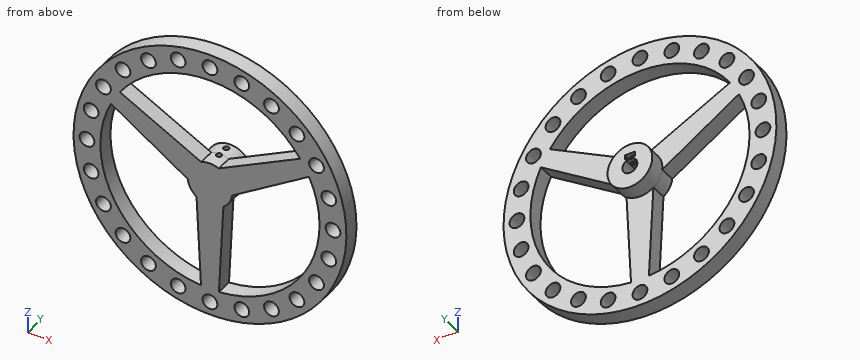
```python
from build123d import *
from build123d.topology import SkipClean

# Parameters (mm, degrees)
SKETCH1_R                      = 76.2
BOSS_EXTRUDE1_DEPTH            = 9
SKETCH2_R                      = 12.5
BOSS_EXTRUDE2_DEPTH            = 9
CUT_EXTRUDE1_DEPTH             = 13
CUT_EXTRUDE2_START             = -1
CUT_EXTRUDE2_DEPTH             = 2.5
CUT_EXTRUDE3_REACH             = 116.376
SKETCH5_R                      = 1.5
CUT_EXTRUDE3_DIRECTION_2_REACH = 116.376
SKETCH6_W                      = 5.5
SKETCH6_H                      = 2.5
CUT_EXTRUDE4_DEPTH             = 109.188743625
SKETCH7_R                      = 4.125
CUT_EXTRUDE5_DEPTH             = 109.138244862
CIRPATTERN1_COUNT              = 24


with BuildPart() as part:
    # Sketch1 → Boss-Extrude1 (new body)
    with BuildSketch(Plane(origin=(0, 0, 0), x_dir=(1, 0, 0), z_dir=(0, 1, 0))):
        with Locations(Location((0, 0, 0), (0, 0, 270))):
            Circle(SKETCH1_R)
        with BuildLine():
            Line((-7.5, 10), (-5, 60.995409663))
            ThreePointArc((-5, 60.995409663), (-53.000754712, 30.6), (-55.323574283, -26.167577813))
            Line((-55.323574283, -26.167577813), (-12.410254038, 1.495190528))
            ThreePointArc((-12.410254038, 1.495190528), (-10.825317547, 6.25), (-7.5, 10))
        make_face(mode=Mode.SUBTRACT)
        with BuildLine():
            Line((5, 60.995409663), (7.5, 10))
            ThreePointArc((7.5, 10), (10.825317547, 6.25), (12.410254038, 1.495190528))
            Line((12.410254038, 1.495190528), (55.323574283, -26.167577813))
            ThreePointArc((55.323574283, -26.167577813), (53.000754712, 30.6), (5, 60.995409663))
        make_face(mode=Mode.SUBTRACT)
        with BuildLine():
            Line((50.323574283, -34.827831851), (4.910254038, -11.495190528))
            ThreePointArc((4.910254038, -11.495190528), (0, -12.5), (-4.910254038, -11.495190528))
            Line((-4.910254038, -11.495190528), (-50.323574283, -34.827831851))
            ThreePointArc((-50.323574283, -34.827831851), (0, -61.2), (50.323574283, -34.827831851))
        make_face(mode=Mode.SUBTRACT)
    extrude(amount=BOSS_EXTRUDE1_DEPTH)

    # Sketch2 → Boss-Extrude2 (add)
    with BuildSketch(Plane(origin=(0, 9, 0), x_dir=(1, 0, 0), z_dir=(0, 1, 0))):
        with Locations(Location((0, 0, 0), (0, 0, 126.869897646))):
            Circle(SKETCH2_R)
    extrude(amount=BOSS_EXTRUDE2_DEPTH)

    # Sketch3 → Cut-Extrude1 (cut)
    with BuildSketch(Plane.XZ.offset(-18)):
        with BuildLine():
            Line((-1.981161276, 3.675), (1.981161276, 3.675))
            ThreePointArc((1.981161276, 3.675), (0, -4.175), (-1.981161276, 3.675))
        make_face()
    extrude(amount=CUT_EXTRUDE1_DEPTH, mode=Mode.SUBTRACT)

    # Sketch4 → Cut-Extrude2 (cut)
    with BuildSketch(Plane(origin=(0, 0, 3.675), x_dir=(-1, 0, 0), z_dir=(0, 0, -1)).offset(CUT_EXTRUDE2_START)):
        Polygon((0, 11.175426481), (-2.75, 9.58771324), (-2.75, 6.41228676), (0, 4.824573519), (2.75, 6.41228676), (2.75, 9.58771324), align=None)
    extrude(amount=-CUT_EXTRUDE2_DEPTH, mode=Mode.SUBTRACT)

    # Sketch5 → Cut-Extrude3 (cut, up to next)
    with BuildSketch(Plane(origin=(0, 0, 7.175), x_dir=(-1, 0, 0), z_dir=(0, 0, -1)), mode=Mode.PRIVATE) as cut_extrude3_sk1:
        with Locations((0, 8)):
            Circle(SKETCH5_R)
    cut_extrude3_tool1 = extrude(cut_extrude3_sk1.sketch, amount=-CUT_EXTRUDE3_REACH, mode=Mode.PRIVATE) & part.part
    # Sketch5 → Cut-Extrude3 (cut, up to next)
    with BuildSketch(Plane(origin=(0, 0, 7.175), x_dir=(-1, 0, 0), z_dir=(0, 0, -1)), mode=Mode.PRIVATE) as cut_extrude3_sk2:
        with Locations((0, 14.5)):
            Circle(SKETCH5_R)
    cut_extrude3_tool2 = extrude(cut_extrude3_sk2.sketch, amount=-CUT_EXTRUDE3_REACH, mode=Mode.PRIVATE) & part.part
    add(cut_extrude3_tool1.solids().sort_by_distance((0, 8, 7.175))[0], mode=Mode.SUBTRACT)
    add(cut_extrude3_tool2.solids().sort_by_distance((0, 14.5, 7.175))[0], mode=Mode.SUBTRACT)

    # Sketch5 → Cut-Extrude3 direction 2 (cut, up to next)
    with BuildSketch(Plane(origin=(0, 0, 7.175), x_dir=(-1, 0, 0), z_dir=(0, 0, -1)), mode=Mode.PRIVATE) as cut_extrude3_direction_2_sk1:
        with Locations((0, 8)):
            Circle(SKETCH5_R)
    cut_extrude3_direction_2_tool1 = extrude(cut_extrude3_direction_2_sk1.sketch, amount=CUT_EXTRUDE3_DIRECTION_2_REACH, mode=Mode.PRIVATE) & part.part
    # Sketch5 → Cut-Extrude3 direction 2 (cut, up to next)
    with BuildSketch(Plane(origin=(0, 0, 7.175), x_dir=(-1, 0, 0), z_dir=(0, 0, -1)), mode=Mode.PRIVATE) as cut_extrude3_direction_2_sk2:
        with Locations((0, 14.5)):
            Circle(SKETCH5_R)
    cut_extrude3_direction_2_tool2 = extrude(cut_extrude3_direction_2_sk2.sketch, amount=CUT_EXTRUDE3_DIRECTION_2_REACH, mode=Mode.PRIVATE) & part.part
    add(cut_extrude3_direction_2_tool1.solids().sort_by_distance((0, 8, 7.175))[0], mode=Mode.SUBTRACT)
    add(cut_extrude3_direction_2_tool2.solids().sort_by_distance((0, 14.5, 7.175))[0], mode=Mode.SUBTRACT)

    # Sketch6 → Cut-Extrude4 (cut, through all)
    with BuildSketch(Plane(origin=(0, 9.58771324, 0), x_dir=(1, 0, 0), z_dir=(0, 1, 0))):
        with Locations((0, -5.925)):
            Rectangle(SKETCH6_W, SKETCH6_H)
    extrude(amount=CUT_EXTRUDE4_DEPTH, mode=Mode.SUBTRACT)

    # Sketch7 → Cut-Extrude5 (cut, through all)
    with SkipClean():  # the faces are left unmerged after this step: merging them gives an invalid solid
        with BuildSketch(Plane(origin=(0, 9, 0), x_dir=(1, 0, 0), z_dir=(0, 1, 0))):
            with Locations(Location((0, 68.7, 0), (0, 0, 270))):
                Circle(SKETCH7_R)
        cut_extrude5 = extrude(amount=-CUT_EXTRUDE5_DEPTH, mode=Mode.SUBTRACT)

    # CirPattern1: Cut-Extrude5 ×24 about axis
    with SkipClean():  # the faces are left unmerged after this step: merging them gives an invalid solid
        cirpattern1_axis = Axis((0, 0, 0), (0, 1, 0))
        for i in range(1, CIRPATTERN1_COUNT):
            add(cut_extrude5.rotate(cirpattern1_axis, i * 360 / CIRPATTERN1_COUNT), mode=Mode.SUBTRACT)


solid = part.part
```
Verification items for the finished model (mm, model axes). Coordinates: 2 decimals unless noted, no trailing zeros. Loops run counter-clockwise (first coordinate to the right, second up) from the corner with the lowest first, then second, coordinate; pieces in that order, holes last. Notation, with made-up numbers: (-37, 7.25) - (16, 7.25) arc R22 cw to (16, 26.25) - close; hole circle Ø6 at (82.5, -23). An arc over 180 degrees is marked (long way). Put each result on its own line as item: value.
Item 1: Section check A-A (x = 34.35). Enter the section's corners in (y, z), then the cut area to 3 significant figures.
Conclusion:
outline: (0, -68.02) - (9, -68.02) - (9, -63.62) - (0, -63.62) - close; (0, -55.37) - (9, -55.37) - (9, -50.65) - (0, -50.65) - close; (0, 12.65) - (9, 12.65) - (9, 26.62) - (0, 26.62) - close; (0, 50.65) - (9, 50.65) - (9, 55.37) - (0, 55.37) - close; (0, 63.62) - (9, 63.62) - (9, 68.02) - (0, 68.02) - close
area: 290 mm2
Item 2: Section check D-D (x = -68.7). Enter the section's corners in (y, z) (3 decimals), then the cut area to 3 significant figures.
Conclusion:
outline: (0, -32.966) - (9, -32.966) - (9, -21.177) - (0, -21.177) - close; (0, -14.384) - (9, -14.384) - (9, -4.125) - (0, -4.125) - close; (0, 4.125) - (9, 4.125) - (9, 14.384) - (0, 14.384) - close; (0, 21.177) - (9, 21.177) - (9, 32.966) - (0, 32.966) - close
area: 397 mm2
Item 3: Section check B-B (z = -34.35). Enter the section's corners in (x, y).
Conclusion:
outline: (-68.02, 0) - (-63.62, 0) - (-63.62, 9) - (-68.02, 9) - close; (-55.37, 0) - (-50.65, 0) - (-50.65, 9) - (-55.37, 9) - close; (-6.31, 0) - (6.31, 0) - (6.31, 9) - (-6.31, 9) - close; (50.65, 0) - (55.37, 0) - (55.37, 9) - (50.65, 9) - close; (63.62, 0) - (68.02, 0) - (68.02, 9) - (63.62, 9) - close
Item 4: Gauge pin test, flat ends, axial feed: pin 1 Ø12 at (x, z) = (31.5, 48.5) entering from -Y; pin 2 Ø7.5 at (x, z) = (34.35, -59.5) entering from +Y; pin 3 Ø4 at (x, y) = (-50, 3.5) entering from +Z; pin 4 Ø0.8 at (y, z) = (10, 6.5) entering from -X. Record the tip position at first contact, or that the pin passes through.
Conclusion:
pin 1: stops at y = 0
pin 2: passes through
pin 3: stops at z = 59.18
pin 4: stops at x = -10.91
Item 5: Scan lines: line 1 along X through (y, z) = (8.5, -33); line 2 along Z through (x, y) = (41, 6); line 3 along X through (y, z) = (6.5, -50). Record each from-to range of solid material in increasing order.
Conclusion:
line 1: x = -68.68 to -63.39, -55.6 to -51.54, -6.37 to 6.37, 51.54 to 55.6, 63.39 to 68.68
line 2: z = -64.23 to -45.44, 16.93 to 30.04, 45.44 to 64.23
line 3: x = -57.5 to -52.45, -44.71 to -35.29, -5.54 to 5.54, 35.29 to 44.71, 52.45 to 57.5
Item 6: Section check C-C (z = -68.7). Enter the section's corners in (x, y) (3 decimals).
Conclusion:
outline: (-32.966, 0) - (-21.177, 0) - (-21.177, 9) - (-32.966, 9) - close; (-14.384, 0) - (-4.125, 0) - (-4.125, 9) - (-14.384, 9) - close; (4.125, 0) - (14.384, 0) - (14.384, 9) - (4.125, 9) - close; (21.177, 0) - (32.966, 0) - (32.966, 9) - (21.177, 9) - close
